The model under review builds one solid part; all positions refer to its coordinate system, in mm. Face numbers are marked on the shaded views. Give positions to 0.01 mm unless a question says otherwise; leave off trailing zeros. Order: outer loops, then holes, each group sorted by start corner. A loop starts at its lowest first (then second) coordinate and runs counter-clockwise, first axis right, second up. Notation, with made-up numbers: (14, 51) - (54, 51) arc R12 ccw to (54, 71) - close; hole circle Ø3 at (24.25, -12.75). An arc over 180 degrees is marked (long way). Use CSV: the item, a comma, the result in double quotes. Start each with the question number.
1. Draft analysis for pull direction Y (two halves, no side actions). For the marked faces 1, 2 and 3, state which applies: released by +Y, released by -Y, zero draft, split by the parting line, or undercut.
2. For pin 1 (1.5 mm diameter, centred on x = -5, y = -2.5, fed in from +Z); pin 2 (8 mm diameter, centred on x = 10.5, z = 8, fed in from +Y); pin 3 (1 mm diameter, centred on x = 6.5, z = 13, fed in from +Y); pin 4 (3 mm diameter, centred on y = -6.5, z = 8.5, fed in from +X), all flat-tipped, find the tip position at first contact; note any pin that passes through.
3. Take a section at A-A, the plane z = 1.25. State the section outline as (x, y) points.
4. To check wall thickness, follow line 1 (Y direction, x = 0, z = 5.75); line 2 (Y direction, x = 1.25, z = 12). State the ranges of each line that lie inside material, in increasing order. Write a range as [from, to].
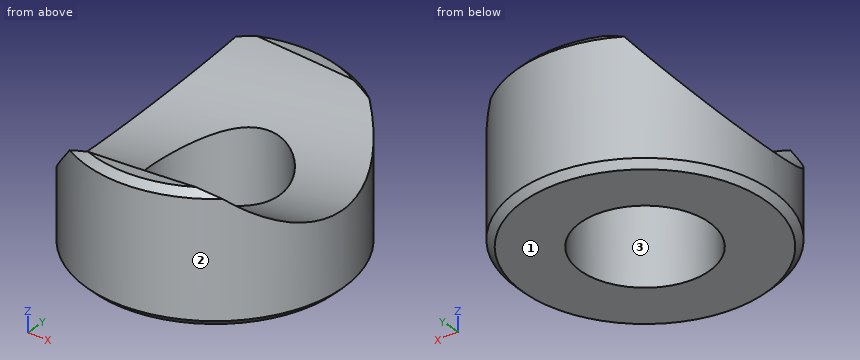
```python
from build123d import *

# Parameters (mm, degrees)
F0_R     = 14.5
F0_R_2   = 7.3
F1_DEPTH = 14.53
F4_SIZE  = 0.762
F5_R     = 14.25
F6_DEPTH = 127


with BuildPart() as f1:
    # F0 (on Top) → F1 (new body)
    with BuildSketch(Plane.XY):
        Circle(F0_R)
        Circle(F0_R_2, mode=Mode.SUBTRACT)
    extrude(amount=F1_DEPTH)

    # F4
    f4_edges = [f1.edges().sort_by_distance(p)[0] for p in [
        (-14.5, 0, 14.53),
        (-14.5, 0, 0),
    ]]
    chamfer(f4_edges, length=F4_SIZE)

    # F5 (on face) → F6 (cut)
    with BuildSketch(Plane(origin=(-13.530054, 0, -1.901525), x_dir=(0, -1, 0), z_dir=(-0.990268, 0, -0.139173))):
        with Locations((0, 21.21935)):
            Circle(F5_R)
    extrude(amount=-F6_DEPTH, mode=Mode.SUBTRACT)


solid = f1.part
```
Determined:
1,face 1,"zero draft"
1,face 2,"split by the parting line"
1,face 3,"undercut"
2,pin 1,"passes through"
2,pin 2,"stops at y = 12.96"
2,pin 3,"stops at y = 13.2"
2,pin 4,"stops at x = 13.61"
3,outline,"circle Ø29 at (0, 0); hole circle Ø14.6 at (0, 0)"
4,line 1,"y = [-14.5, -7.3], [7.3, 14.5]"
4,line 2,"y = [-14.45, -10.61], [10.61, 14.45]"
